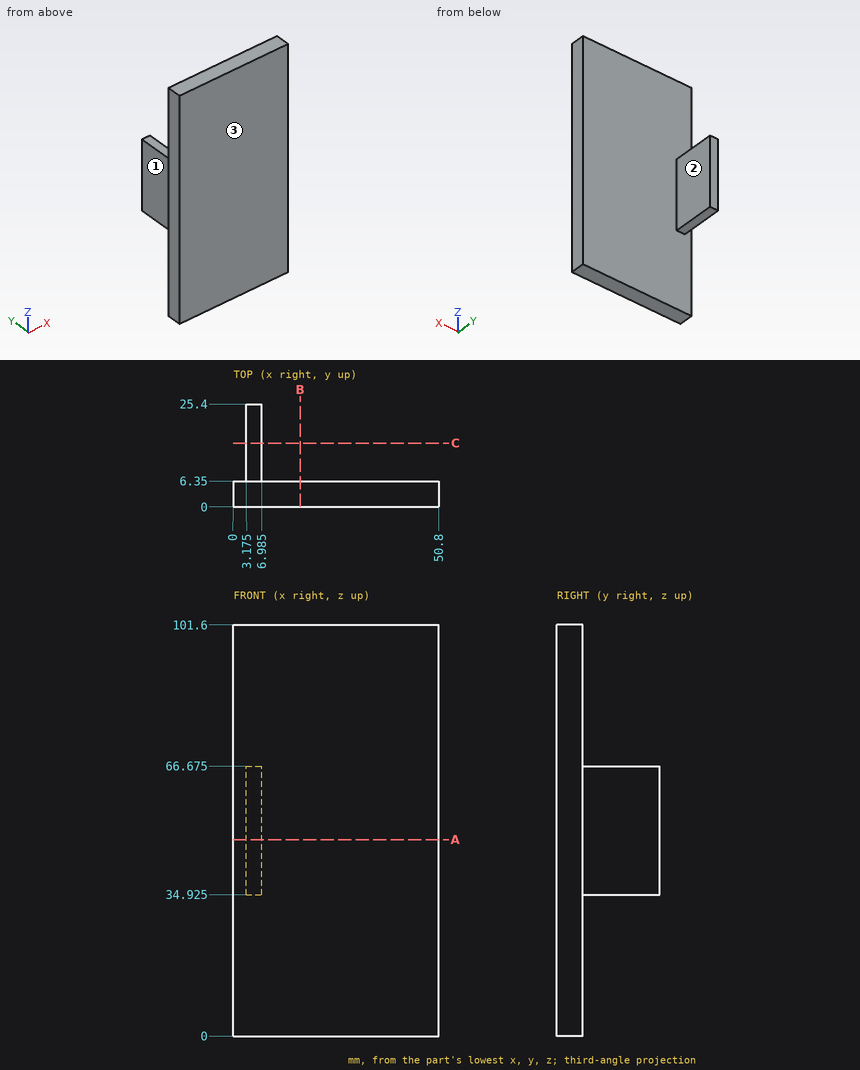
Study the drawing (mm; zero at the part's minimum x, y, z) and answer. A direction names the side the tool comes from. Give positions to 0.01 mm unless a question says otherwise; leave off trailing zeros. Loops run counter-clockwise (first coordinate to the right, second up) from the corner with the lowest first, then second, coordinate; pieces in that order, holes last. Notation, with made-up numbers: (45, -33.75) - (60, -33.75) arc R27 cw to (60, -10.75) - close; hole circle Ø7 at (49.25, 42.25). An arc over 180 degrees is marked (long way). One line per question, with ' | ' between items.
(1) Straight lines are drawn through the part: probe 1 along Y at (x, z) = (24.5, 80); probe 2 along X at (y, z) = (13.5, 56.5) (3 decimals); probe 3 along Z at (x, y) = (4, 11.75) (3 decimals). For each, find the intervals that lie inside material, in ascending order.
Recorded:
probe 1: y = 0 to 6.35 | probe 2: x = 3.175 to 6.985 | probe 3: z = 34.925 to 66.675
(2) The part is cut by section C-C (y = 15.75). Write down the section's boundary in (x, z) (3 decimals).
Recorded:
outline: (3.175, 34.925) - (6.985, 34.925) - (6.985, 66.675) - (3.175, 66.675) - close
(3) The part is cut by section A-A (z = 48.5). Write down the section's boundary in (x, y) (3 decimals), then the cut area to 3 significant figures.
Recorded:
outline: (0, 0) - (50.8, 0) - (50.8, 6.35) - (6.985, 6.35) - (6.985, 25.4) - (3.175, 25.4) - (3.175, 6.35) - (0, 6.35) - close | area: 395 mm²
(4) A tool of negligible diameter and unlimited length cuts with its end or side. For the marked faces 1, 2 and 3, from which of +Z, -Z, +X, -X, +Y, -Y can it reach the whole face along a straight path? Write none if from no direction.
Recorded:
face 1: +Z, -Z, -X, +Y | face 2: +Z, -Z, +X, +Y | face 3: +Z, -Z, +X, -X, -Y
(5) The part is cut by section B-B (x = 16.5). Write down the section's boundary in (y, z), then the cut area to 3 significant figures.
Recorded:
outline: (0, 0) - (6.35, 0) - (6.35, 101.6) - (0, 101.6) - close | area: 645 mm²
(6) Each of these flat-tipped pins is pushed along its axis until it touches: pin 1 Ø1.5 at (y, z) = (13, 61.5) entering from +X (3 decimals); pin 2 Ø15 at (y, z) = (20.5, 55) entering from -X (3 decimals); pin 3 Ø8 at (x, y) = (9, 12.5) entering from +Z (3 decimals); pin 4 Ø2 at (x, z) = (34, 59) entering from -Y. Where does it stop, or does it pass through?
Recorded:
pin 1: stops at x = 6.985 | pin 2: stops at x = 3.175 | pin 3: stops at z = 66.675 | pin 4: stops at y = 0
